Verification items for the finished model (mm, model axes). A direction names the side the tool comes from. Coordinates: 2 decimals unless noted, no trailing zeros. Write each loop counter-clockwise with the first axis right and the second up, starting at its lowest first coordinate (ties: lowest second). Pieces come first, ordered by that corner, then holes. Notation, with made-up numbers: (72.25, -32) -> (130.25, -32) arc R18 ccw to (130.25, -7) -> close; hole circle Ø11 at (-33.75, -24.75). An arc over 180 degrees is marked (long way). Answer in a Markdown table with one row per item.
Autodesk Inventor part; units mm, degrees
ref_plane "YZ Plane" through (0, 0, 0) normal (1, 0, 0) x (0, 1, 0)
ref_plane "XZ Plane" through (0, 0, 0) normal (0, 1, 0) x (-1, 0, 0)
ref_plane "XY Plane" through (0, 0, 0) normal (0, 0, 1) x (1, 0, 0)
sketch "Sketch1" plane through (0, 0, 0) normal (0, 0, 1) x (1, 0, 0)
  circle A0 centre (0, 0) radius 3.175
  line L0 (-3.175, 0) -> (-3.175, -165.1)
  line L1 (3.175, 0) -> (3.175, -165.1)
  line L2 (-3.175, -165.1) -> (3.175, -165.1)
  dimension "d0" = 6.35
  dimension "d1" = 165.1
  dimension "d2" = 165.1
extrude "Extrusion1" add sketch "Sketch1" along normal blind 6.35
sketch "Sketch2" plane through (0, 0, 6.35) normal (0, 0, 1) x (1, 0, 0)
  circle A0 centre (0, 0) radius 3.175
  dimension "d5" = 6.35
extrude "Extrusion2" add sketch "Sketch2" along normal blind 31.75
sketch "Sketch3" plane through (0, 0, 0) normal (0, 0, -1) x (-1, 0, 0)
  circle A0 centre (0, 0) radius 3.175
  dimension "d8" = 6.35
extrude "Extrusion3" add sketch "Sketch3" along normal blind 31.75
sketch "Sketch5" plane through (3.175, -165.1, 0) normal (1, 0, 0) x (0, 0, -1)
  circle A0 centre (-3.175, 3.175) radius 1.5875
  circle A1 centre (-3.175, 9.525) radius 1.5875
  circle A2 centre (-3.175, 15.875) radius 1.5875
  line L0 (-6.35, 0) -> (-6.35, 165.1)
  line L1 (0, 0) -> (-6.35, 0)
  point P0 (0, 165.1)
  dimension "d11" = 3.175
  dimension "d12" = 3.175
  dimension "d13" = 3.175
  dimension "d14" = 3.175
  dimension "d15" = 3.175
  dimension "d16" = 6.35
  dimension "d17" = 6.35
extrude "Extrusion4" cut sketch "Sketch5" against normal blind 12.7
properties part number "PendulumHanger"
1. Go/stop test with flat-tipped pins: pin 1 (3.5 mm diameter, centred on y = -161.925, z = 3.175, fed in from -X) (3 decimals); pin 2 (2 mm diameter, centred on x = -1.5, z = -19, fed in from -Y); pin 3 (1 mm diameter, centred on x = 1, y = -19.5, fed in from +Z). Record where each tip stops, or that it passes through.
Findings below:
| item | result |
|---|---|
| pin 1 | stops at x = -3.175 |
| pin 2 | stops at y = -3.14 |
| pin 3 | stops at z = 6.35 |
2. Sectioned sample at B-B, the plane z = 12.5. Record the cut outline in (x, y) (3 decimals), and give its area (3 significant figures).
Findings below:
| item | result |
|---|---|
| outline | circle Ø6.35 at (0, 0) |
| area | 31.7 mm² |
3. Release check for a two-part mould opening along Z. For faces 3 (the face through (0.044, -150.775, 3.519)), 4 (the face through (0, 0, 38.1)), 5 (the face through (3.175, -81, 3)) record: released by +Z, released by -Z, zero draft, split by the parting line, or undercut.
Findings below:
| item | result |
|---|---|
| face 3 | undercut |
| face 4 | released by +Z |
| face 5 | zero draft |
4. Material ranges on probe 1 along Z at (x, y) = (-2, -88); probe 2 along Y at (x, z) = (0.25, 29); probe 3 along Y at (x, z) = (2.5, -19.5), recorded low to high. Write a range as from..to.
Findings below:
| item | result |
|---|---|
| probe 1 | z = 0..6.35 |
| probe 2 | y = -3.17..3.17 |
| probe 3 | y = -1.96..1.96 |
5. Access from +Z, -Z, +X, -X, +Y, -Y to the whole of each face (thin tool, end or side, straight path). Record for faces 1 (the face through (0, -165.1, 3)), 2 (the face through (2.639, 1.765, 2.686)).
Findings below:
| item | result |
|---|---|
| face 1 | +Z, -Z, +X, -X, -Y |
| face 2 | none |
6. Sectioned sample at C-C, the plane y = -109.5. Record the cut outline in (x, z) (3 decimals), and give its area (3 significant figures).
Findings below:
| item | result |
|---|---|
| outline | (-3.175, 0) -> (3.175, 0) -> (3.175, 6.35) -> (-3.175, 6.35) -> close |
| area | 40.3 mm² |
7. Sectioned sample at A-A, the plane x = 1.75. Count the separate pieces of the cut face and the enclosed holes in it, and give its area (3 significant figures).
Findings below:
| item | result |
|---|---|
| separate pieces | 1 |
| enclosed holes | 3 |
| area | 1,380 mm² |
